Geometry: final body of the model. Coordinates: model frame, mm. Face numbers are marked on the shaded views. Give positions to 0.01 mm unless a question says otherwise; leave off trailing zeros. Loops run counter-clockwise (first coordinate to the right, second up) from the corner with the lowest first, then second, coordinate; pieces in that order, holes last.
```python
from build123d import *

# Parameters (mm, degrees)
SKETCH2_R               = 7.5
BOSS_EXTRUDE1_DEPTH     = 0.1
SKETCH3_R               = 1
CUT_EXTRUDE2_DEPTH      = 11.607073112
FILL_PATTERN3_OUTLINE_R = 1
FILL_PATTERN3_DEPTH     = 0.1
SKETCH5_R               = 7.874751998
SKETCH5_R_2             = 7
BOSS_EXTRUDE2_DEPTH     = 0.1


# Read off the part's stored shape, not the designer's step: Fill Pattern3
with BuildPart() as part:
    # Sketch2 → Boss-Extrude1 (new body)
    with BuildSketch(Plane(origin=(0, 0, 0), x_dir=(1, 0, 0), z_dir=(0, 1, 0))):
        with Locations(Location((0, 0, 0), (0, 0, 270))):
            Circle(SKETCH2_R)
    extrude(amount=BOSS_EXTRUDE1_DEPTH)

    # Sketch3 → Cut-Extrude2 (cut, through all)
    with BuildSketch(Plane(origin=(0, 0, 0), x_dir=(1, 0, 0), z_dir=(0, 1, 0))):
        with Locations(Location((0, 0, 0), (0, 0, 270))):
            Circle(SKETCH3_R)
    extrude(amount=CUT_EXTRUDE2_DEPTH, mode=Mode.SUBTRACT)

    # Fill Pattern3 outline → Fill Pattern3 (cut)
    with BuildSketch(Plane(origin=(0, 0, 0), x_dir=(1, 0, 0), z_dir=(0, 1, 0))):
        with Locations((3, -3)):
            Circle(FILL_PATTERN3_OUTLINE_R)
        with Locations((0, -3)):
            Circle(FILL_PATTERN3_OUTLINE_R)
        with Locations((-3, -3)):
            Circle(FILL_PATTERN3_OUTLINE_R)
        with Locations((-3, 0)):
            Circle(FILL_PATTERN3_OUTLINE_R)
        with Locations((-3, 3)):
            Circle(FILL_PATTERN3_OUTLINE_R)
        with Locations((0, 3)):
            Circle(FILL_PATTERN3_OUTLINE_R)
        with Locations((6, 0)):
            Circle(FILL_PATTERN3_OUTLINE_R)
        with Locations((0, 6)):
            Circle(FILL_PATTERN3_OUTLINE_R)
        with Locations((-6, 0)):
            Circle(FILL_PATTERN3_OUTLINE_R)
        with Locations((0, -6)):
            Circle(FILL_PATTERN3_OUTLINE_R)
        with Locations((3, 0)):
            Circle(FILL_PATTERN3_OUTLINE_R)
        with Locations((3, 3)):
            Circle(FILL_PATTERN3_OUTLINE_R)
    extrude(amount=FILL_PATTERN3_DEPTH, mode=Mode.SUBTRACT)

    # Sketch5 → Boss-Extrude2 (add)
    with BuildSketch(Plane(origin=(0, 0, 0), x_dir=(1, 0, 0), z_dir=(0, 1, 0))):
        with Locations(Location((0, 0, 0), (0, 0, 270))):
            Circle(SKETCH5_R)
        with Locations(Location((0, 0, 0), (0, 0, 270))):
            Circle(SKETCH5_R_2, mode=Mode.SUBTRACT)
    extrude(amount=-BOSS_EXTRUDE2_DEPTH)


solid = part.part
```
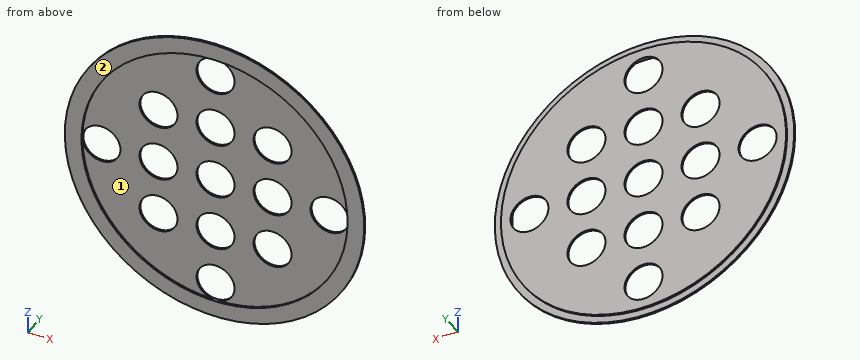
Q1. Section query D-D, the plane x = 6. Return loops of the section in (y, z).
Q2. Section query A-A, the plane x = 3.75. Return loops of the section in (y, z), and give its area (3 significant figures).
Q3. Section query B-B, the plane y = 0.05. State how many separate pieces and enclosed holes the cut face has, and give its area (3 significant figures).
Q4. Material intervals for probe 1 along X at (y, z) = (0.05, 0); probe 2 along X at (y, z) = (-0.05, -0.25); probe 3 along Z at (x, y) = (-3, 0.05), sorted ascending.
Q5. Mould query, pull axis Z, two halves, no side actions, for the marked faces 1 and 2. Classes: +Z half, -Z half, draft (parallel to the pull), parting line (faces both ways), or undercut.
Q6. Pin query (flat end, axial travel): pin 1 Ø2.5 at (x, z) = (3, -3) entering from -Y. Return the tip coordinate at first contact, or that it passes through.
Q7. Section query C-C, the plane z = 5.5. Return loops of the section in (x, y), and give its area (3 significant figures).
Resolved:
1. outline: (-0.1, -5.1) - (0, -5.1) - (0, -4.5) - (0.1, -4.5) - (0.1, -1) - (0, -1) - (0, -3.61) - (-0.1, -3.61) - close; (-0.1, 3.61) - (0, 3.61) - (0, 1) - (0.1, 1) - (0.1, 4.5) - (0, 4.5) - (0, 5.1) - (-0.1, 5.1) - close
2. outline: (-0.1, -6.92) - (0, -6.92) - (0, -6.5) - (0.1, -6.5) - (0.1, -3.66) - (0, -3.66) - (0, -5.91) - (-0.1, -5.91) - close; (-0.1, 5.91) - (0, 5.91) - (0, 3.66) - (0.1, 3.66) - (0.1, 6.5) - (0, 6.5) - (0, 6.92) - (-0.1, 6.92) - close; (0, -2.34) - (0.1, -2.34) - (0.1, -0.66) - (0, -0.66) - close; (0, 0.66) - (0.1, 0.66) - (0.1, 2.34) - (0, 2.34) - close
2. area: 1.10 mm2
3. separate pieces: 1
3. enclosed holes: 13
3. area: 136 mm2
4. probe 1: x = -7.5 to -7, -5 to -4, -2 to -1, 1 to 2, 4 to 5, 7 to 7.5
4. probe 2: x = -7.87 to -7, 7 to 7.87
4. probe 3: z = -6.87 to -4, -2 to -1, 1 to 2, 4 to 6.87
5. face 1: undercut
5. face 2: draft
6. pin 1: stops at y = 0
7. outline: (-5.64, -0.1) - (-4.33, -0.1) - (-4.33, 0) - (-0.87, 0) - (-0.87, 0.1) - (-5.1, 0.1) - (-5.1, 0) - (-5.64, 0) - close; (0.87, 0) - (4.33, 0) - (4.33, -0.1) - (5.64, -0.1) - (5.64, 0) - (5.1, 0) - (5.1, 0.1) - (0.87, 0.1) - close
7. area: 1.11 mm2
